from build123d import *

# Parameters (mm, degrees)
SKETCH1_W           = 25
SKETCH1_H           = 25
SKETCH1_R           = 2.15
BOSS_EXTRUDE1_DEPTH = 1.5875


with BuildPart() as part:
    # Sketch1 → Boss-Extrude1 (new body, symmetric)
    with BuildSketch(Plane(origin=(0, 0, 0), x_dir=(1, 0, 0), z_dir=(0, 1, 0))):
        Rectangle(SKETCH1_W, SKETCH1_H)
        with Locations((-8, 8)):
            Circle(SKETCH1_R, mode=Mode.SUBTRACT)
        with Locations((8, 8)):
            Circle(SKETCH1_R, mode=Mode.SUBTRACT)
        with Locations((8, -8)):
            Circle(SKETCH1_R, mode=Mode.SUBTRACT)
        with Locations((-8, -8)):
            Circle(SKETCH1_R, mode=Mode.SUBTRACT)
        Polygon((-2.749630657, -4.7625), (2.749630657, -4.7625), (5.499261314, 0), (2.749630657, 4.7625), (-2.749630657, 4.7625), (-5.499261314, 0), align=None, mode=Mode.SUBTRACT)
    extrude(amount=BOSS_EXTRUDE1_DEPTH, both=True)


solid = part.part
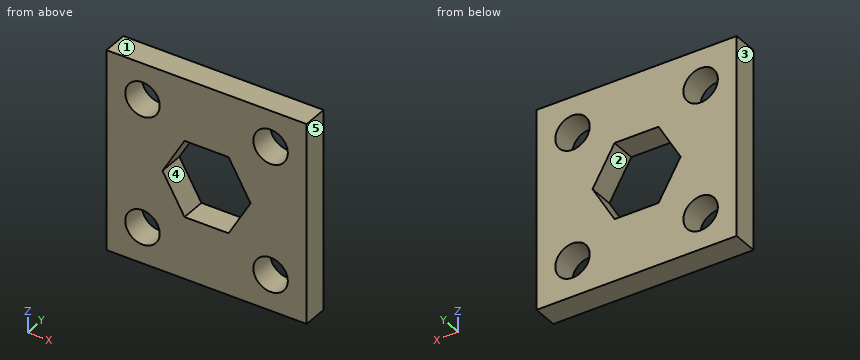
Geometry: final body of the model. Coordinates: model frame, mm. Face numbers are marked on the shaded views. A direction names the side the tool comes from. Give positions to 0.01 mm unless a question says otherwise; leave off trailing zeros. Loops run counter-clockwise (first coordinate to the right, second up) from the corner with the lowest first, then second, coordinate; pieces in that order, holes last. Notation, with made-up numbers: (47.25, 64.5) - (64.25, 64.5) arc R20 cw to (64.25, 73.5) - close; hole circle Ø5 at (38, 17.5). An arc over 180 degrees is marked (long way). Answer as CSV lines item,"result". Start each with the question number.
1. Draft query along Z for the marked faces 1, 2 and 3. Return one class per face: released by +Z, released by -Z, zero draft, split by the parting line, or undercut.
2. Section B-B, the plane x = 8. Return loops of the section in (y, z).
3. Section C-C, the plane z = 8. Return loops of the section in (x, y), plus the area to 3 significant figures.
4. Pin query (flat end, axial travel): P1, Ø4, axis at x = 8, z = 8, coming from the -Y side. Return the tip coordinate at first contact, or that it passes through.
5. Reachability of the marked faces 4 and 5 from +Z, -Z, +X, -X, +Y, -Y: full face, straight path, thin tool, end or side. Return the list, or none.
6. Ray query, L1, parallel to X at y = -0.7, z = 8; L2, parallel to Z at x = 0.5, y = -1. Return the intervals inside material, ascending.
7. Section A-A, the plane y = -1. Return loops of the section in (x, z), plus the area to 3 significant figures.
Answers:
1,face 1,"released by +Z"
1,face 2,"undercut"
1,face 3,"zero draft"
2,outline,"(-1.59, -12.5) - (1.59, -12.5) - (1.59, -10.15) - (-1.59, -10.15) - close; (-1.59, -5.85) - (1.59, -5.85) - (1.59, 5.85) - (-1.59, 5.85) - close; (-1.59, 10.15) - (1.59, 10.15) - (1.59, 12.5) - (-1.59, 12.5) - close"
3,outline,"(-12.5, -1.59) - (-10.15, -1.59) - (-10.15, 1.59) - (-12.5, 1.59) - close; (-5.85, -1.59) - (5.85, -1.59) - (5.85, 1.59) - (-5.85, 1.59) - close; (10.15, -1.59) - (12.5, -1.59) - (12.5, 1.59) - (10.15, 1.59) - close"
3,area,"52.1 mm2"
4,P1,"passes through"
5,face 4,"+Y, -Y"
5,face 5,"+Z, -Z, +X, +Y, -Y"
6,L1,"x = -12.5 to -10.15, -5.85 to 5.85, 10.15 to 12.5"
6,L2,"z = -12.5 to -4.76, 4.76 to 12.5"
7,outline,"(-12.5, -12.5) - (12.5, -12.5) - (12.5, 12.5) - (-12.5, 12.5) - close; hole circle Ø4.3 at (-8, -8); hole circle Ø4.3 at (-8, 8); hole (-5.5, 0) - (-2.75, -4.76) - (2.75, -4.76) - (5.5, 0) - (2.75, 4.76) - (-2.75, 4.76) - close; hole circle Ø4.3 at (8, -8); hole circle Ø4.3 at (8, 8)"
7,area,"488 mm2"
